Geometry: see drawing. Coordinates: mm, zero at the bounding-box minimum. Coordinates: 2 decimals unless noted, no trailing zeros. Order: outer loops, then holes, each group sorted by start corner. A loop starts at its lowest first (then second) coordinate and runs counter-clockwise, first axis right, second up.
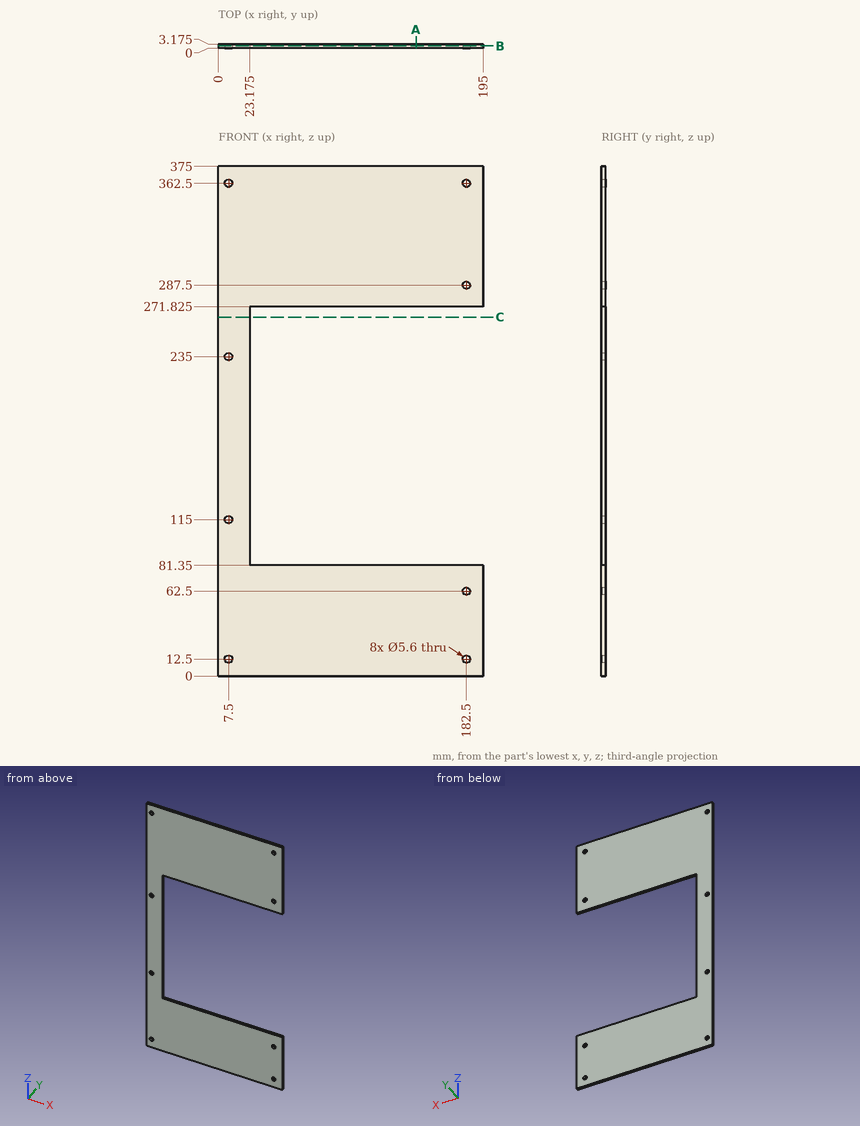
Q1. Material intervals for line 1 along X through (y, z) = (1.9, 12.5); line 2 along Z through (x, y) = (178, 0.9) (3 decimals); line 3 along X through (y, z) = (1, 235) (3 decimals), sorted ascending.
Solutions:
line 1: x = 0 to 4.7, 10.3 to 179.7, 185.3 to 195
line 2: z = 0 to 81.35, 271.825 to 375
line 3: x = 0 to 4.7, 10.3 to 23.175
Q2. Section query A-A on x = 145.5. Output: boundary loops of the cut face in (y, z) (3 decimals), plus the area to 3 significant figures.
Solutions:
outline: (0, 0) - (3.175, 0) - (3.175, 81.35) - (0, 81.35) - close; (0, 271.825) - (3.175, 271.825) - (3.175, 375) - (0, 375) - close
area: 586 mm2
Q3. Pin query (flat end, axial travel): P1, Ø5, axis at x = 7.5, z = 12.5, coming from the -Y side; P2, Ø1, axis at y = 1, z = 137, coming from the +X side (3 decimals). Return the tip coordinate at first contact, or that it passes through.
Solutions:
P1: passes through
P2: stops at x = 23.175
Q4. Section query C-C on z = 264. Output: boundary loops of the cut face in (x, y) (3 decimals).
Solutions:
outline: (0, 0) - (23.175, 0) - (23.175, 3.175) - (0, 3.175) - close
Q5. Section query B-B on y = 1.85. Give the number of separate pieces and of enclosed holes in the cut face, plus the area to 3 significant figures.
Solutions:
separate pieces: 1
enclosed holes: 8
area: 40,200 mm2
